Geometry: final body of the model. Coordinates: model frame, mm. Face numbers are marked on the shaded views. A direction names the side the tool comes from. Round coordinates to 2 decimals unless told otherwise and drop trailing zeros. Loops run counter-clockwise (first coordinate to the right, second up) from the corner with the lowest first, then second, coordinate; pieces in that order, holes last. Notation, with made-up numbers: (19.25, 18) -> (31.25, 18) arc R18 cw to (31.25, 46) -> close; hole circle Ø4 at (-2.5, -35). An arc over 180 degrees is marked (long way). Answer in a Markdown table with one row per item.
```python
from build123d import *

# Parameters (mm, degrees)
SKETCH1_W           = 25.4
SKETCH1_H           = 101.6
BOSS_EXTRUDE1_DEPTH = 25.4
SKETCH2_R           = 3.175
CUT_EXTRUDE1_DEPTH  = 59.198711326
BOSS_EXTRUDE2_DEPTH = 25.4
SKETCH4_W           = 20.32
SKETCH4_H           = 12.7
CUT_EXTRUDE2_DEPTH  = 152.4


with BuildPart() as part:
    # Sketch1 → Boss-Extrude1 (new body)
    with BuildSketch(Plane(origin=(0, 0, 0), x_dir=(1, 0, 0), z_dir=(0, 1, 0))):
        Rectangle(SKETCH1_W, SKETCH1_H)
    extrude(amount=BOSS_EXTRUDE1_DEPTH)

    # Sketch2 → Cut-Extrude1 (cut, through all)
    with BuildSketch(Plane(origin=(0, 25.4, 0), x_dir=(1, 0, 0), z_dir=(0, 1, 0))):
        with Locations(Location((0, -25.480397296, 0), (0, 0, 270))):
            Circle(SKETCH2_R)
        with BuildLine():
            Line((3.175, 44.369602704), (3.175, 6.269602704))
            ThreePointArc((3.175, 6.269602704), (0, 3.094602704), (-3.175, 6.269602704))
            Line((-3.175, 6.269602704), (-3.175, 44.369602704))
            ThreePointArc((-3.175, 44.369602704), (0, 47.544602704), (3.175, 44.369602704))
        make_face()
    extrude(amount=-CUT_EXTRUDE1_DEPTH, mode=Mode.SUBTRACT)

    # Sketch3 → Boss-Extrude2 (add)
    with BuildSketch(Plane(origin=(0, 0, 0), x_dir=(1, 0, 0), z_dir=(0, 1, 0))):
        Polygon((-12.7, 50.8), (-12.7, 91.44), (38.196727149, 91.44), (38.196727149, 72.39), (0, 72.39), (0, 54.61), (12.7, 54.61), (12.7, 50.8), align=None)
    extrude(amount=BOSS_EXTRUDE2_DEPTH)

    # Sketch4 → Cut-Extrude2 (cut)
    with BuildSketch(Plane(origin=(0, 25.4, 0), x_dir=(1, 0, 0), z_dir=(0, 1, 0))):
        with Locations((14.387739516, 78.74)):
            Rectangle(SKETCH4_W, SKETCH4_H)
    extrude(amount=-CUT_EXTRUDE2_DEPTH, mode=Mode.SUBTRACT)


solid = part.part
```
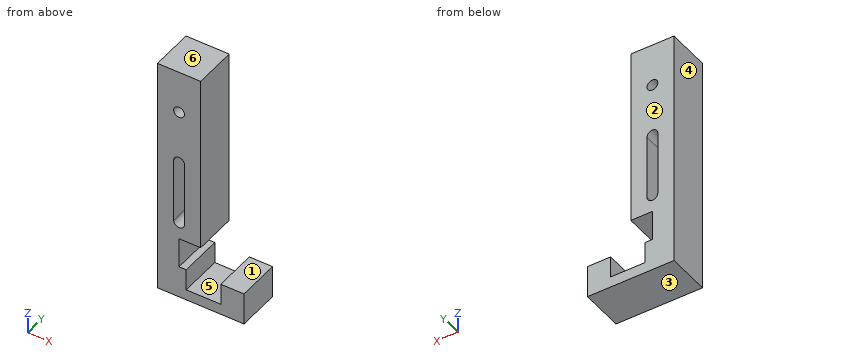
Item 1: First-contact query: P1, Ø11, axis at x = 34.5, y = 8.5, coming from the +Z side; P2, Ø2, axis at y = 12.5, z = -41, coming from the +X side; P3, Ø5.5, axis at y = 8.5, z = -66.5, coming from the +X side. Flat tips, straight axial feed; report the tip coordinate or a pass-through.
Ans:
| item | result |
|---|---|
| P1 | z = -72.39 |
| P2 | x = 12.7 |
| P3 | x = 0 |
Item 2: Section query B-B, the plane y = 18.25. Output: boundary loops of the cut face in (x, z) (3 decimals), and give its area (3 significant figures).
Ans:
| item | result |
|---|---|
| outline | (-12.7, -91.44) -> (38.197, -91.44) -> (38.197, -72.39) -> (24.548, -72.39) -> (24.548, -85.09) -> (4.228, -85.09) -> (4.228, -72.39) -> (0, -72.39) -> (0, -54.61) -> (12.7, -54.61) -> (12.7, 50.8) -> (-12.7, 50.8) -> close; hole (-3.175, -44.37) arc R3.175 ccw to (3.175, -44.37) -> (3.175, -6.27) arc R3.175 ccw to (-3.175, -6.27) -> close; hole circle Ø6.35 at (0, 25.48) |
| area | 3,310 mm2 |
Item 3: Section query D-D, the plane x = 20. Output: boundary loops of the cut face in (y, z).
Ans:
| item | result |
|---|---|
| outline | (0, -91.44) -> (25.4, -91.44) -> (25.4, -85.09) -> (0, -85.09) -> close |
Item 4: Mould query, pull axis Z, two halves, no side actions, for the marked faces 3, 4, 5 and 6. Classes: released by +Z, released by -Z, zero draft, split by the parting line, or undercut.
Ans:
| item | result |
|---|---|
| face 3 | released by -Z |
| face 4 | zero draft |
| face 5 | undercut |
| face 6 | released by +Z |
Item 5: Section query C-C, the plane x = 6. Output: boundary loops of the cut face in (y, z).
Ans:
| item | result |
|---|---|
| outline | (0, -91.44) -> (25.4, -91.44) -> (25.4, -85.09) -> (0, -85.09) -> close; (0, -54.61) -> (25.4, -54.61) -> (25.4, 50.8) -> (0, 50.8) -> close |
Item 6: Section query A-A, the plane z = -79.5. Output: boundary loops of the cut face in (x, y), and give its area (3 significant figures).
Ans:
| item | result |
|---|---|
| outline | (-12.7, 0) -> (4.23, 0) -> (4.23, 25.4) -> (-12.7, 25.4) -> close; (24.55, 0) -> (38.2, 0) -> (38.2, 25.4) -> (24.55, 25.4) -> close |
| area | 777 mm2 |
Item 7: Set-up query: the marked faces 1 and 2. Return all of +Z, -Z, +X, -X, +Y, -Y with unobstructed straight access to the full face (end or side cutting, diameter ignored); none if empty.
Ans:
| item | result |
|---|---|
| face 1 | +Z, +X, +Y, -Y |
| face 2 | +Z, -Z, +X, -X, +Y |
Item 8: Ray query, L1, parallel to Z at x = -2, y = 13; L2, parallel to X at y = 10.75, z = -30 (3 decimals); L3, parallel to X at y = 21, z = -75.5. Return the intervals inside material, ascending.
Ans:
| item | result |
|---|---|
| L1 | -91.44 to -46.84, -3.8 to 23.01, 27.95 to 50.8 |
| L2 | -12.7 to -3.175, 3.175 to 12.7 |
| L3 | -12.7 to 4.23, 24.55 to 38.2 |
